Check sheet for the modelled part. Datum: model origin and axes. Units: mm. A direction names the side the tool comes from. Round coordinates to 2 decimals unless told otherwise and drop trailing zeros. Order: outer loops, then holes, each group sorted by start corner. A loop starts at its lowest first (then second) coordinate and runs counter-clockwise, first axis right, second up.
(1) Mould release check, pull along Y, two halves, no side actions. Record for faces 1 (the flat face through (14, 76.555, 58)), 2 (the cylindrical face through (-15.361, 3.104, 27.083)), 3 (the flat face through (-14, 101.955, 41)), 4 (the flat face through (40.258, 89.077, 40.519)): released by +Y, released by -Y, zero draft, split by the parting line, or undercut.
(2) Sectioned sample at C-C, the plane x = 65. Enter the section's corners in (y, z).
(3) Thickness scan on probe 1 along Y at (x, z) = (-40.5, 40); probe 2 along Z at (x, y) = (-14.5, 45); probe 3 along Z at (x, y) = (-10, 0). Record the ranges inside material, lowest first.
(4) Sectioned sample at A-A, the plane y = 0. Enter the section's corners in (x, z).
(5) Sectioned sample at D-D, the plane y = -36. Enter the section's corners in (x, z).
(6) Tool access check on faces 5 (the flat face through (-42, 1, 76.2)), 6 (the flat face through (34.64, -18.08, 38.63)), 7 (the flat face through (-18, -76.555, 29)). Record the directions out of +Z, -Z, +X, -X, +Y, -Y that give a thin tool (end or side, any length) a straight path to the whole face; none if there is none.
(7) Sectioned sample at B-B, the plane z = 33.5. Enter the section's corners in (x, y).
(8) Depth check by flat-ended pin: pin 1 (1.5 mm diameter, centred on x = 61.5, y = 81, fed in from +Z); pin 2 (1.5 mm diameter, centred on x = -2, y = 21, fed in from +Z); pin 3 (10 mm diameter, centred on y = 56, z = 41, fed in from +X); pin 4 (5 mm diameter, centred on x = 33, y = 78, fed in from -Z). Enter the tip coordinate at first touch or a pass-through.
```python
from build123d import *

# Parameters (mm, degrees)
F0_W     = 153.8918465376
F0_H     = 153.1105190516
F1_DEPTH = 76.2
F3_DEPTH = 254
F4_R     = 14.3164019678
F5_DEPTH = 508
F7_DEPTH = 25.4
F9_DEPTH = 63.5


with BuildPart() as f1:
    # F0 (on Top) → F1 (new body)
    with BuildSketch(Plane.XY):
        Rectangle(F0_W, F0_H)
    extrude(amount=F1_DEPTH)

    # F2 (on face) → F3 (cut, symmetric)
    with BuildSketch(Plane.XZ.offset(76.5552595258)):
        Polygon((76.9459232688, 76.2), (-6.5071131103, 76.2), (76.9459232688, 0), align=None)
    extrude(amount=F3_DEPTH, both=True, mode=Mode.SUBTRACT)

    # F4 (on face) → F5 (cut)
    with BuildSketch(Plane(origin=(-76.9459232688, 0, 0), x_dir=(0, -1, 0), z_dir=(-1, 0, 0))):
        with Locations((0, 41.0589724779)):
            Circle(F4_R)
    extrude(amount=-F5_DEPTH, mode=Mode.SUBTRACT)

    # F6 (on face) → F7 (join)
    with BuildSketch(Plane(origin=(0, 76.5552595258, 0), x_dir=(-1, 0, 0), z_dir=(0, 1, 0))):
        Polygon((-81.6596895456, 0), (-76.9459232688, 0), (6.5071131103, 76.2), (76.9459232688, 76.2), (76.9459232688, 79.9183472991), (-81.6596895456, 79.9183472991), align=None)
        Polygon((-76.9459232688, 0), (76.9459232688, 0), (76.9459232688, 76.2), (6.5071131103, 76.2), align=None)
    extrude(amount=F7_DEPTH)

    # F8 (on face) → F9 (cut, symmetric)
    with BuildSketch(Plane.XZ.offset(-76.5552595258)):
        Polygon((0, 79.9183472991), (81.6596895456, 0), (81.6596895456, 79.9183472991), align=None)
    extrude(amount=F9_DEPTH, both=True, mode=Mode.SUBTRACT)


solid = f1.part
```
Derived:
1. face 1: released by -Y
1. face 2: undercut
1. face 3: released by +Y
1. face 4: zero draft
2. outline: (-76.56, 0) - (101.96, 0) - (101.96, 16.3) - (76.56, 16.3) - (76.56, 10.91) - (-76.56, 10.91) - close
3. probe 1: y = -76.56 to -14.28, 14.28 to 101.96
3. probe 2: z = 0 to 76.2
3. probe 3: z = 0 to 26.74, 55.38 to 76.2
4. outline: (-76.95, 0) - (76.95, 0) - (47.66, 26.74) - (-76.95, 26.74) - close; (-76.95, 55.38) - (16.3, 55.38) - (-6.51, 76.2) - (-76.95, 76.2) - close
5. outline: (-76.95, 0) - (76.95, 0) - (-6.51, 76.2) - (-76.95, 76.2) - close
6. face 5: +Z, +X, -X, -Y
6. face 6: +Z, +X, -Y
6. face 7: +Z, -Z, +X, -X, -Y
7. outline: (-76.95, -76.56) - (40.26, -76.56) - (40.26, -12.16) - (-76.95, -12.16) - close; (-76.95, 12.16) - (40.26, 12.16) - (40.26, 76.56) - (47.43, 76.56) - (47.43, 101.96) - (-76.95, 101.96) - close
8. pin 1: stops at z = 20.46
8. pin 2: stops at z = 72.77
8. pin 3: stops at x = 37.52
8. pin 4: stops at z = 0
